For this review, use the dimensioned drawing (mm, ordinates from the lowest corner) and the shaded views. Coordinates: 2 decimals unless noted, no trailing zeros. Write each loop counter-clockwise with the first axis right and the second up, starting at its lowest first coordinate (ties: lowest second). Pieces come first, ordered by that corner, then holes. Notation, with made-up numbers: (24, 32.5) - (34, 32.5) arc R19 ccw to (34, 54.5) - close; hole circle Ø11 at (85.5, 52.5). An arc over 180 degrees is marked (long way). Put each result on its own line as item: value.
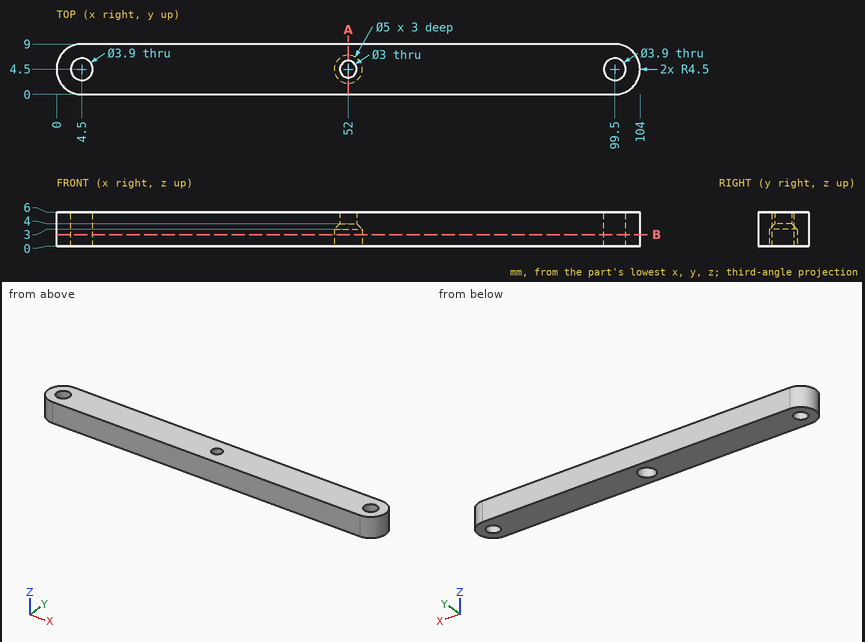
1. Consider section B-B on z = 2.05. State the section outline as (x, y) points, plus the area to 3 significant figures.
Determined:
outline: (4.5, 0) - (99.5, 0) arc R4.5 ccw to (99.5, 9) - (4.5, 9) arc R4.5 ccw to start; hole circle Ø3.9 at (4.5, 4.5); hole circle Ø5 at (52, 4.5); hole circle Ø3.9 at (99.5, 4.5)
area: 875 mm^2
2. To check wall thickness, follow probe 1 along Y at (x, z) = (52, 5); probe 2 along Y at (x, z) = (4.5, 4.4); probe 3 along X at (y, z) = (5.5, 1.9). State the ranges of each line that lie inside material, in increasing order.
Determined:
probe 1: y = 0 to 3, 6 to 9
probe 2: y = 0 to 2.55, 6.45 to 9
probe 3: x = 0.11 to 2.83, 6.17 to 49.71, 54.29 to 97.83, 101.17 to 103.89
3. Consider section A-A on x = 52. State the section outline as (y, z) points, plus the area to 3 significant figures.
Determined:
outline: (0, 0) - (2, 0) - (2, 3) - (3, 4) - (3, 6) - (0, 6) - close; (6, 4) - (7, 3) - (7, 0) - (9, 0) - (9, 6) - (6, 6) - close
area: 29.0 mm^2
4. For pin 1 Ø2 at (y, z) = (3.5, 2.5) entering from +X; pin 2 Ø4 at (x, y) = (52, 4.5) entering from -Z, all flat-tipped, find the tip position at first contact; note any pin that passes through.
Determined:
pin 1: stops at x = 104
pin 2: stops at z = 3.5
